from build123d import *

# Parameters (mm, degrees)
SKETCH1_R              = 105
BOSS_EXTRUDE1_DEPTH    = 75
SKETCH3_R              = 105
SKETCH3_R_2            = 65
CUT_EXTRUDE1_DEPTH     = 5
CUT_EXTRUDE2_REACH     = 92
CUT_EXTRUDE2_START     = -15
SKETCH4_R              = 105
SKETCH4_R_2            = 70
SKETCH5_R              = 55.4
CUT_EXTRUDE3_DEPTH     = 32.5
SKETCH6_R              = 55
CUT_EXTRUDE4_DEPTH     = 20
CUT_EXTRUDE5_REACH     = 24.5
SKETCH7_R              = 50
F_12_0MM_DOWEL_HOLE1_D = 13
F_6_0MM_DOWEL_HOLE1_D  = 7


with BuildPart() as part:
    # Sketch1 → Boss-Extrude1 (new body)
    with BuildSketch(Plane(origin=(0, 0, 0), x_dir=(1, 0, 0), z_dir=(0, 1, 0))):
        Circle(SKETCH1_R)
    extrude(amount=BOSS_EXTRUDE1_DEPTH)

    # Sketch3 → Cut-Extrude1 (cut)
    with BuildSketch(Plane.XZ):
        Circle(SKETCH3_R)
        Circle(SKETCH3_R_2, mode=Mode.SUBTRACT)
    extrude(amount=-CUT_EXTRUDE1_DEPTH, mode=Mode.SUBTRACT)

    # Sketch4 → Cut-Extrude2 (cut, up to next)
    with BuildSketch(Plane.XZ.offset(CUT_EXTRUDE2_START), mode=Mode.PRIVATE) as cut_extrude2_sk1:
        Circle(SKETCH4_R)
        Circle(SKETCH4_R_2, mode=Mode.SUBTRACT)
    cut_extrude2_tool1 = extrude(cut_extrude2_sk1.sketch, amount=-CUT_EXTRUDE2_REACH, mode=Mode.PRIVATE) & part.part
    add(cut_extrude2_tool1.solids().sort_by_distance((-102.030152, 15, 0))[0], mode=Mode.SUBTRACT)

    # Sketch5 → Cut-Extrude3 (cut)
    with BuildSketch(Plane.XZ):
        Circle(SKETCH5_R)
    extrude(amount=-CUT_EXTRUDE3_DEPTH, mode=Mode.SUBTRACT)

    # Sketch6 → Cut-Extrude4 (cut)
    with BuildSketch(Plane.XZ.offset(-32.5)):
        Circle(SKETCH6_R)
    extrude(amount=-CUT_EXTRUDE4_DEPTH, mode=Mode.SUBTRACT)

    # Sketch7 → Cut-Extrude5 (cut, up to next)
    with BuildSketch(Plane.XZ.offset(-52.5), mode=Mode.PRIVATE) as cut_extrude5_sk1:
        Circle(SKETCH7_R)
    cut_extrude5_tool1 = extrude(cut_extrude5_sk1.sketch, amount=-CUT_EXTRUDE5_REACH, mode=Mode.PRIVATE) & part.part
    add(cut_extrude5_tool1.solids().sort_by_distance((0, 52.5, 0))[0], mode=Mode.SUBTRACT)

    # Ø12.0mm Dowel Hole1 (through all)
    with Locations(Plane(origin=(0, 15, 0), x_dir=(1, 0, 0), z_dir=(0, 1, 0))):
        with Locations((45, 77.942286341), (90, 0), (45, -77.942286341), (-45, -77.942286341), (-90, 0), (-45, 77.942286341)):
            Hole(F_12_0MM_DOWEL_HOLE1_D / 2)

    # Ø6.0mm Dowel Hole1 (through all)
    with Locations(Plane(origin=(0, 75, 0), x_dir=(1, 0, 0), z_dir=(0, 1, 0))):
        with Locations((-62.5, 0), (0, 62.5), (62.5, 0), (0, -62.5)):
            Hole(F_6_0MM_DOWEL_HOLE1_D / 2)


solid = part.part
Geometry: final body of the model. Coordinates: model frame, mm. A direction names the side the tool comes from. Round coordinates to 2 decimals unless told otherwise and drop trailing zeros. Loops run counter-clockwise (first coordinate to the right, second up) from the corner with the lowest first, then second, coordinate; pieces in that order, holes last.
Q1. Section B-B on x = 43. State how many separate pieces and enclosed holes the cut face has, plus the area to 3 significant figures.
Q2. Section D-D on z = -75. Return loops of the section in (x, y), plus the area to 3 significant figures.
Q3. Access query for faces 1 (the flat face through (12, 52.5, -49)), 2 (the cylindrical face through (-55.55, 44.58, -42.594)), 3 (the cylindrical face through (0, 37, 59)). Directions: +Z, -Z, +X, -X, +Y, -Y. A direction counts if a zero-diameter tool reaches every point of the face in a straight line with its end or side. Return the directions, or none.
Q4. Pin query (flat end, axial travel): P1, Ø6, axis at x = -8.5, z = 84, coming from the +Y side; P2, Ø3, axis at x = 74.5, z = -4.5, coming from the -Y side; P3, Ø10.5, axis at x = -45, z = 77.94, coming from the -Y side; P4, Ø8, axis at x = 28, y = 66.5, coming from the -Z side. Return the tip coordinate at first contact, or that it passes through.
Q5. Material intervals for L1, parallel to Z at x = 0, y = 63.5; L2, parallel to Z at x = 2.5, y = 63; L3, parallel to Y at x = -71, z = 23, sorted ascending.
Q6. Section C-C on y = 23.5. Return loops of the section in (x, z).
Q7. Section A-A on z = 62.5. Return loops of the section in (x, y), plus the area to 3 significant figures.
Q8. Pull-direction query (X, two-part tool) for faces 4 (the cylindrical face through (-45.48, 2.46, 46.44)), 5 (the cylindrical face through (46.44, 2.46, 45.48)), 6 (the cylindrical face through (46.409, 9.93, -71.597)), 7 (the cylindrical face through (-43.591, 9.93, 84.288)); classes: released by +X, released by -X, zero draft, split by the parting line, or undercut.
Evaluation:
1. separate pieces: 4
1. enclosed holes: 0
1. area: 3,990 mm2
2. outline: (-73.48, 5) - (-50.8, 5) - (-50.8, 15) - (-73.48, 15) - close; (-39.2, 5) - (39.2, 5) - (39.2, 15) - (-39.2, 15) - close; (50.8, 5) - (73.48, 5) - (73.48, 15) - (50.8, 15) - close
2. area: 1,240 mm2
3. face 1: -Y
3. face 2: +Y
3. face 3: +Y, -Y
4. P1: stops at y = 15
4. P2: stops at y = 5
4. P3: passes through
4. P4: stops at z = -65.76
5. L1: z = -70 to -66, -59 to -50, 50 to 59, 66 to 70
5. L2: z = -69.96 to -64.95, -60.05 to -49.94, 49.94 to 60.05, 64.95 to 69.96
5. L3: y = 5 to 15
6. outline: circle Ø140 at (0, 0); hole circle Ø7 at (-62.5, 0); hole circle Ø110.8 at (0, 0); hole circle Ø7 at (0, -62.5); hole circle Ø7 at (0, 62.5); hole circle Ø7 at (62.5, 0)
7. outline: (-84.37, 5) - (-17.85, 5) - (-17.85, 0) - (-3.5, 0) - (-3.5, 75) - (-31.52, 75) - (-31.52, 15) - (-84.37, 15) - close; (3.5, 0) - (17.85, 0) - (17.85, 5) - (84.37, 5) - (84.37, 15) - (31.52, 15) - (31.52, 75) - (3.5, 75) - close
7. area: 5,120 mm2
8. face 4: released by -X
8. face 5: released by +X
8. face 6: undercut
8. face 7: undercut
